from build123d import *

# Parameters (mm, degrees)
BOSS_EXTRUDE1_DEPTH = 5
SKETCH1_3_R         = 5
BOSS_EXTRUDE2_DEPTH = 10


with BuildPart() as part:
    # Sketch1 → Boss-Extrude1 (new body)
    with BuildSketch(Plane.XY):
        with BuildLine():
            Line((70.64516129, -15), (-66.903225806, -15))
            ThreePointArc((-66.903225806, -15), (-81.903225806, 0), (-66.903225806, 15))
            Line((-66.903225806, 15), (70.64516129, 15))
            ThreePointArc((70.64516129, 15), (85.64516129, 0), (70.64516129, -15))
        make_face()
        with BuildLine():
            Line((-66.903225806, -10), (50.64516129, -10))
            ThreePointArc((50.64516129, -10), (60.64516129, 0), (50.64516129, 10))
            Line((50.64516129, 10), (-66.903225806, 10))
            ThreePointArc((-66.903225806, 10), (-76.903225806, 0), (-66.903225806, -10))
        make_face(mode=Mode.SUBTRACT)
    extrude(amount=BOSS_EXTRUDE1_DEPTH)

    # Sketch1_3 → Boss-Extrude2 (add)
    with BuildSketch(Plane.XY):
        with Locations((70.64516129, 0)):
            Circle(SKETCH1_3_R)
    extrude(amount=-BOSS_EXTRUDE2_DEPTH)


solid = part.part
Source: CAD feature listing. Evaluate the final solid. Frame: model axes, mm. A direction names the side the tool comes from. Give positions to 0.01 mm unless a question says otherwise; leave off trailing zeros. Order: outer loops, then holes, each group sorted by start corner. A loop starts at its lowest first (then second) coordinate and runs counter-clockwise, first axis right, second up. Notation, with made-up numbers: (55.25, 75) -> (61.25, 75) arc R19 ccw to (61.25, 82) -> close; hole circle Ø2 at (73.25, 89.5). An arc over 180 degrees is marked (long way). Write item = value, one per line.
Item 1: Mould query, pull axis X, two halves, no side actions, for faces 1 (the face through (21.7, 10.2, 5)), 2 (the face through (60.643, -0.22, 2.465)), 3 (the face through (-7, 10, 2)), 4 (the face through (-81.9, -0.3, 2.5)). Classes: +X half, -X half, draft (parallel to the pull), parting line (faces both ways), or undercut.
Check result:
face_1 = draft
face_2 = undercut
face_3 = undercut
face_4 = -X half
Item 2: Ray query, probe 1 along Y at (x, z) = (-56.5, 2.5); probe 2 along Z at (x, y) = (61.5, 12); probe 3 along X at (y, z) = (5.5, 3.5). Return the intervals inside material, ascending.
Check result:
probe_1 = -15 to -10, 10 to 15
probe_2 = 0 to 5
probe_3 = -80.86 to -75.25, 59 to 84.6
Item 3: Section query D-D (x = 55.5). Output: boundary loops of the cut face in (y, z).
Check result:
outline = (-15, 0) -> (-8.74, 0) -> (-8.74, 5) -> (-15, 5) -> close; (8.74, 0) -> (15, 0) -> (15, 5) -> (8.74, 5) -> close
Item 4: Section query A-A (x = 3). Output: boundary loops of the cut face in (y, z), then the cut area to 3 significant figures.
Check result:
outline = (-15, 0) -> (-10, 0) -> (-10, 5) -> (-15, 5) -> close; (10, 0) -> (15, 0) -> (15, 5) -> (10, 5) -> close
area = 50.0 mm²
Item 5: Section query C-C (z = -4.25). Output: boundary loops of the cut face in (x, y), then the cut area to 3 significant figures.
Check result:
outline = circle Ø10 at (70.65, 0)
area = 78.5 mm²
Item 6: Contact query for a flat-ended pin moving along its axis: pin 1 (6 mm diameter, centred on y = 7.5, z = -6, fed in from -X). Output: stop coordinate, or through.
Check result:
pin_1 = 68.47
Item 7: Section query B-B (y = 0). Output: boundary loops of the cut face in (x, z).
Check result:
outline = (-81.9, 0) -> (-76.9, 0) -> (-76.9, 5) -> (-81.9, 5) -> close; (60.65, 0) -> (65.65, 0) -> (65.65, -10) -> (75.65, -10) -> (75.65, 0) -> (85.65, 0) -> (85.65, 5) -> (60.65, 5) -> close
Item 8: Set-up query: faces 5 (the face through (1, 15, 2)), 6 (the face through (-9, -10, 2)), 7 (the face through (75.26, -1.92, -4.93)). Return all of +Z, -Z, +X, -X, +Y, -Y with unobstructed straight access to the full face (end or side cutting, diameter ignored); none if empty.
Check result:
face_5 = +Z, -Z, +X, -X, +Y
face_6 = +Z, -Z
face_7 = -Z
